```python
from build123d import *

# Parameters (mm, degrees)
SKETCH_1_R          = 0.65
SKETCH_1_R_2        = 1.5
EXTRUDE_1_DEPTH     = 2.3
SKETCH_2_R          = 4.4
EXTRUDE_2_DEPTH     = 3.2
SKETCH_3_R          = 4.4
SKETCH_3_R_2        = 3.4
SKETCH_3_R_3        = 2.75
SKETCH_3_R_4        = 1.5
CUT_EXTRUDE_1_DEPTH = 1
CUT_EXTRUDE1_REACH  = 22.67


with BuildPart() as part:
    # Эскиз1 → Бобышка-Вытянуть1 (new body)
    with BuildSketch(Plane.XY):
        with BuildLine():
            Line((-3.968626967, 4.5), (-16.888114198, 2.469689731))
            ThreePointArc((-16.888114198, 2.469689731), (-19, 0), (-16.888114198, -2.469689731))
            Line((-16.888114198, -2.469689731), (-3.968626967, -4.5))
            ThreePointArc((-3.968626967, -4.5), (0, -6), (3.968626967, -4.5))
            Line((3.968626967, -4.5), (16.888114198, -2.469689731))
            ThreePointArc((16.888114198, -2.469689731), (19, 0), (16.888114198, 2.469689731))
            Line((16.888114198, 2.469689731), (3.968626967, 4.5))
            ThreePointArc((3.968626967, 4.5), (0, 6), (-3.968626967, 4.5))
        make_face()
        with Locations((-16.5, 0)):
            Circle(SKETCH_1_R, mode=Mode.SUBTRACT)
        with Locations((-13.5, 0)):
            Circle(SKETCH_1_R, mode=Mode.SUBTRACT)
        with Locations((-10.5, 0)):
            Circle(SKETCH_1_R, mode=Mode.SUBTRACT)
        with Locations((-7.5, 0)):
            Circle(SKETCH_1_R, mode=Mode.SUBTRACT)
        with Locations(Location((16.5, 0, 0), (0, 0, 180))):
            Circle(SKETCH_1_R, mode=Mode.SUBTRACT)
        with Locations(Location((7.5, 0, 0), (0, 0, 180))):
            Circle(SKETCH_1_R, mode=Mode.SUBTRACT)
        with Locations(Location((10.5, 0, 0), (0, 0, 180))):
            Circle(SKETCH_1_R, mode=Mode.SUBTRACT)
        with Locations(Location((13.5, 0, 0), (0, 0, 180))):
            Circle(SKETCH_1_R, mode=Mode.SUBTRACT)
        Circle(SKETCH_1_R_2, mode=Mode.SUBTRACT)
    extrude(amount=EXTRUDE_1_DEPTH)

    # Эскиз2 → Бобышка-Вытянуть2 (add)
    with BuildSketch(Plane.XY.offset(2.3)):
        with Locations(Location((0, 0, 0), (0, 0, 180))):
            Circle(SKETCH_2_R)
        Polygon((0.333439775, 2.639447604), (0, 3.05), (-0.333439775, 2.639447604), (-0.758504156, 2.954178641), (-0.979368078, 2.473601404), (-1.469348706, 2.672735374), (-1.563759083, 2.15232973), (-2.087868673, 2.223354314), (-2.049893354, 1.695819264), (-2.575200173, 1.634271725), (-2.407225286, 1.132754236), (-2.900722375, 0.942501833), (-2.6133024, 0.498514094), (-3.043981522, 0.191511085), (-2.655176114, -0.167049522), (-2.995976115, -0.571513009), (-2.530215347, -0.822116802), (-2.75972251, -1.298626839), (-2.246271844, -1.42552746), (-2.35006539, -1.944143169), (-1.821186821, -1.939366985), (-1.792745019, -2.467501833), (-1.281669931, -2.33134895), (-1.122779886, -2.835818282), (-0.661621006, -2.576843686), (-0.382266362, -3.025949839), (0, -2.660425857), (0.382266362, -3.025949839), (0.661621006, -2.576843686), (1.122779886, -2.835818282), (1.281669931, -2.33134895), (1.792745019, -2.467501833), (1.821186821, -1.939366985), (2.35006539, -1.944143169), (2.246271844, -1.42552746), (2.75972251, -1.298626839), (2.530215347, -0.822116802), (2.995976115, -0.571513009), (2.655176114, -0.167049522), (3.043981522, 0.191511085), (2.6133024, 0.498514094), (2.900722375, 0.942501833), (2.407225286, 1.132754236), (2.575200173, 1.634271725), (2.049893354, 1.695819264), (2.087868673, 2.223354314), (1.563759083, 2.15232973), (1.469348706, 2.672735374), (0.979368078, 2.473601404), (0.758504156, 2.954178641), align=None, mode=Mode.SUBTRACT)
    extrude(amount=EXTRUDE_2_DEPTH)

    # Эскиз3 → Вырез-Вытянуть1 (cut)
    # profile 1 of 2: a face of its own
    with BuildSketch(Plane(origin=(0, 0, 0), x_dir=(-1, 0, 0), z_dir=(0, 0, -1))):
        Circle(SKETCH_3_R)
        Circle(SKETCH_3_R_2, mode=Mode.SUBTRACT)
    # profile 2 of 2: a face of its own
    with BuildSketch(Plane(origin=(0, 0, 0), x_dir=(-1, 0, 0), z_dir=(0, 0, -1))):
        Circle(SKETCH_3_R_3)
        Circle(SKETCH_3_R_4, mode=Mode.SUBTRACT)
    extrude(amount=-CUT_EXTRUDE_1_DEPTH, mode=Mode.SUBTRACT)

    # Sketch1 → Cut-Extrude1 (cut, up to next)
    with BuildSketch(Plane(origin=(0, 0, 0), x_dir=(-1, 0, 0), z_dir=(0, 0, -1)), mode=Mode.PRIVATE) as cut_extrude1_sk1:
        with BuildLine():
            Line((-3.968626967, 4.5), (-16.888114198, 2.469689731))
            ThreePointArc((-16.888114198, 2.469689731), (-19, 0), (-16.888114198, -2.469689731))
            Line((-16.888114198, -2.469689731), (-3.968626967, -4.5))
            ThreePointArc((-3.968626967, -4.5), (-6, 0), (-3.968626967, 4.5))
        make_face()
    cut_extrude1_tool1 = extrude(cut_extrude1_sk1.sketch, amount=-CUT_EXTRUDE1_REACH, mode=Mode.PRIVATE) & part.part
    add(cut_extrude1_tool1.solids().sort_by_distance((11.282562, 0, 0))[0], mode=Mode.SUBTRACT)


solid = part.part
```
Verification items for the finished model (mm, model axes). A direction names the side the tool comes from. Round coordinates to 2 decimals unless told otherwise and drop trailing zeros. Write each loop counter-clockwise with the first axis right and the second up, starting at its lowest first coordinate (ties: lowest second). Pieces come first, ordered by that corner, then holes. Notation, with made-up numbers: (-8, 66) -> (50, 66) arc R8 ccw to (50, 74) -> close; hole circle Ø2 at (86.5, 48.25). An arc over 180 degrees is marked (long way). Write each question's results on one line, items separated by ' | '.
Q1. Thickness scan on probe 1 along Y at (x, z) = (-16.5, 0.5); probe 2 along Y at (x, z) = (0, 2.05); probe 3 along Z at (x, y) = (-13, -1.5). Record the ranges inside material, lowest first.
Derived:
probe 1: y = -2.53 to -0.65, 0.65 to 2.53 | probe 2: y = -6 to -1.5, 1.5 to 6 | probe 3: z = 0 to 2.3
Q2. Sectioned sample at B-B, the plane x = -10.5. Record the boundary of the cut face in (y, z).
Derived:
outline: (-3.47, 0) -> (-0.65, 0) -> (-0.65, 2.3) -> (-3.47, 2.3) -> close; (0.65, 0) -> (3.47, 0) -> (3.47, 2.3) -> (0.65, 2.3) -> close
Q3. Access from +Z, -Z, +X, -X, +Y, -Y to the whole of each face (thin tool, end or side, straight path). Record for faces 1 (the face through (-1.4, 1.4, 2.3)), 2 (the face through (0.596, -2.685, 0.493)), 3 (the face through (-1.5, 0.07, 1.64)).
Derived:
face 1: +Z | face 2: -Z | face 3: +Z, -Z
Q4. Sectioned sample at C-C, the plane x = -7.5. Record the boundary of the cut face in (y, z).
Derived:
outline: (-3.95, 0) -> (-0.65, 0) -> (-0.65, 2.3) -> (-3.95, 2.3) -> close; (0.65, 0) -> (3.95, 0) -> (3.95, 2.3) -> (0.65, 2.3) -> close
Q5. Sectioned sample at A-A, the plane z = 0.55. Record the boundary of the cut face in (x, y).
Derived:
outline: (-16.89, -2.47) -> (-3.97, -4.5) arc R6 ccw (long way) to (-3.97, 4.5) -> (-16.89, 2.47) arc R2.5 ccw to start; circle Ø6.8 at (0, 0); hole circle Ø1.3 at (-16.5, 0); hole circle Ø1.3 at (-13.5, 0); hole circle Ø1.3 at (-10.5, 0); hole circle Ø1.3 at (-7.5, 0); hole circle Ø8.8 at (0, 0); hole circle Ø5.5 at (0, 0)
Q6. Draft check along Y on faces 4 (the face through (-19, 0, 1)), 5 (the face through (-10.34, 3.5, 1.13)), 6 (the face through (0.74, -3.32, 0.49)). Enter one of: released by +Y, released by -Y, zero draft, split by the parting line, or undercut.
Derived:
face 4: split by the parting line | face 5: released by +Y | face 6: undercut
Q7. Go/stop test with flat-tipped pins: pin 1 Ø2 at (x, y) = (-7.5, 0) entering from +Z; pin 2 Ø2 at (x, z) = (-6, 2) entering from +Y; pin 3 Ø1.5 at (x, z) = (-15, 0.5) entering from +Y. Record where each tip stops, or that it passes through.
Derived:
pin 1: stops at z = 2.3 | pin 2: stops at y = 4.34 | pin 3: stops at y = 2.88
Q8. Sectioned sample at D-D, the plane y = 4.75. Record the boundary of the cut face in (x, z), and give its area (3 significant figures).
Derived:
outline: (-3.67, 0) -> (3.67, 0) -> (3.67, 2.3) -> (-3.67, 2.3) -> close | area: 16.9 mm²
